Geometry check sheet. Reference: the model listing, model coordinates, mm. A direction names the side the tool comes from. Give positions to 0.01 mm unless a question says otherwise; leave off trailing zeros. Loops run counter-clockwise (first coordinate to the right, second up) from the corner with the lowest first, then second, coordinate; pieces in that order, holes last. Notation, with made-up numbers: (82, 30) -> (120, 30) arc R22 ccw to (120, 42) -> close; hole circle Ø7 at (3, 73.25). An arc over 180 degrees is marked (long way). One line per question, with ' | ' between items.
from build123d import *

# Parameters (mm, degrees)
F0_W      = 42
F0_H      = 42
F1_DEPTH  = 8
F2_DEPTH  = 24
F3_DEPTH  = 8
F4_SIZE   = 2.5
F4_2_SIZE = 2.5
F5_SIZE   = 5.5
F7_R      = 11
F7_R_2    = 4
F8_DEPTH  = 1.5
F9_R      = 2.5
F10_DEPTH = 23.5
F12_R     = 0.1


# Not quite as in the source:
# - a feature names something its author has since deleted; it is built from what else it names


with BuildPart() as f1:
    # F0 (on Top) → F1 (new body)
    with BuildSketch(Plane.XY):
        Rectangle(F0_W, F0_H)
    extrude(amount=F1_DEPTH)


with BuildPart() as f2:
    # F2 (new): a face of the model
    f2_faces = [f1.part.faces().sort_by_distance(p)[0] for p in [
        (0, 0, 8),
    ]]
    extrude(f2_faces, amount=F2_DEPTH)


with BuildPart() as f3:
    # F3 (new): a face of the model
    f3_faces = [f2.part.faces().sort_by_distance(p)[0] for p in [
        (0, 0, 32),
    ]]
    extrude(f3_faces, amount=F3_DEPTH)

    # F4#2
    f4_2_edges = [f3.edges().sort_by_distance(p)[0] for p in [
        (-21, -21, 36),
        (-21, 21, 36),
        (21, 21, 36),
        (21, -21, 36),
    ]]
    chamfer(f4_2_edges, length=F4_2_SIZE)

    # F7 (on face) → F8 (join)
    with BuildSketch(Plane.XY.offset(40)):
        Circle(F7_R)
        Circle(F7_R_2, mode=Mode.SUBTRACT)
    extrude(amount=F8_DEPTH)

    # F9 (on face) → F10 (join)
    with BuildSketch(Plane.XY.offset(40)):
        Circle(F9_R)
    extrude(amount=F10_DEPTH)


with BuildPart() as f1_1:
    add(f1.part)

    # F4
    f4_edges = [f1_1.edges().sort_by_distance(p)[0] for p in [
        (-21, -21, 4),
        (-21, 21, 4),
        (21, 21, 4),
        (21, -21, 4),
    ]]
    chamfer(f4_edges, length=F4_SIZE)


with BuildPart() as f2_1:
    add(f2.part)

    # F5
    f5_edges = [f2_1.edges().sort_by_distance(p)[0] for p in [
        (21, -21, 20),
        (-21, -21, 20),
        (-21, 21, 20),
        (21, 21, 20),
    ]]
    chamfer(f5_edges, length=F5_SIZE)


with BuildPart() as f1_2:
    add(f1_1.part)

    # F11: union F2, F3
    add(f2_1.part)
    add(f3.part)

    # F12
    f12_edges = [f1_2.edges().sort_by_distance(p)[0] for p in [
        (11, 0, 40.75),
        (-11, 0, 40),
        (-11, 0, 41.5),
    ]]
    fillet(f12_edges, radius=F12_R)


solid = f1_2.part
Item 1: Release check for a two-part mould opening along Y. For faces 6 (the face through (18.3, -18.2, 19.8)), 7 (the face through (-0.867, -3.905, 40.74)), 8 (the face through (19.7, 19.8, 3.9)) record: pulls with the +Y half, pulls with the -Y half, needs draft (parallel to the pull), parting line crosses it, or undercut.
Result:
face 6: pulls with the -Y half | face 7: undercut | face 8: pulls with the +Y half
Item 2: Sectioned sample at A-A (y = 0). Record the cut outline in (x, z).
Result:
outline: (-21, 0) -> (21, 0) -> (21, 40) -> (11.1, 40) arc R0.1 cw to (11, 40.1) -> (11, 41.4) arc R0.1 ccw to (10.9, 41.5) -> (4, 41.5) -> (4, 40) -> (2.5, 40) -> (2.5, 63.5) -> (-2.5, 63.5) -> (-2.5, 40) -> (-4, 40) -> (-4, 41.5) -> (-10.9, 41.5) arc R0.1 ccw to (-11, 41.4) -> (-11, 40.1) arc R0.1 cw to (-11.1, 40) -> (-21, 40) -> close
Item 3: Sectioned sample at C-C (z = 30.5). Record the cut outline in (x, y), plus the area to 3 significant figures.
Result:
outline: (-21, -15.5) -> (-15.5, -21) -> (15.5, -21) -> (21, -15.5) -> (21, 15.5) -> (15.5, 21) -> (-15.5, 21) -> (-21, 15.5) -> close | area: 1,700 mm2
Item 4: Scan lines: probe 1 along Y at (x, z) = (0, 40.5); probe 2 along Z at (x, y) = (-4.5, -14); probe 3 along Z at (x, y) = (-10, 4). Record each from-to range of solid material in increasing order.
Result:
probe 1: -11 to -4, -2.5 to 2.5, 4 to 11 | probe 2: 0 to 40 | probe 3: 0 to 41.5
Item 5: Sectioned sample at D-D (x = 14). Record the cut outline in (y, z).
Result:
outline: (-21, 0) -> (21, 0) -> (21, 40) -> (-21, 40) -> close
Item 6: Depth check by flat-ended pin: pin 1 Ø1.6 at (x, y) = (17, -17.5) entering from +Z; pin 2 Ø8 at (x, y) = (13, 3.5) entering from +Z. Enter the tip coordinate at first touch or a pass-through.
Result:
pin 1: z = 40 | pin 2: z = 41.5
Item 7: Set-up check for faces 1 (the face through (-19, -19, 32)), 2 (the face through (19, -19, 8)), 3 (the face through (-0.54, -2.44, 51.59)), 4 (the face through (19, 19, 8)), 5 (the face through (-19.7, -19.8, 35.9)): record each of +Z, -Z, +X, -X, +Y, -Y from which the full face is reachable in a straight line by a thin tool's end or side.
Result:
face 1: -X, -Y | face 2: +X, -Y | face 3: +Z | face 4: +X, +Y | face 5: +Z, -Z, -X, -Y
